Source: CAD feature listing. Evaluate the final solid. Frame: model axes, mm. A direction names the side the tool comes from. Round coordinates to 2 decimals unless told otherwise and drop trailing zeros. Loops run counter-clockwise (first coordinate to the right, second up) from the corner with the lowest first, then second, coordinate; pieces in that order, holes last.
Item 1: Access query for faces 1 (the flat face through (-9.2, 0, -11.938)), 2 (the flat face through (-8.7, 0, 0)), 3 (the flat face through (-0.039, 10, 1)), 4 (the flat face through (-5, 0, 11.43)). Directions: +Z, -Z, +X, -X, +Y, -Y. A direction counts if a zero-diameter tool reaches every point of the face in a straight line with its end or side. Return the directions, or none.
Item 2: Section query C-C on y = -6.5. Return loops of the section in (x, z).
Item 3: Section query A-A on z = 7. Return loops of the section in (x, y), then the cut area to 3 significant figures.
Item 4: Ray query, L1, parallel to Y at x = 0, z = 12.3 (3 decimals); L2, parallel to X at y = 0, z = 1.25 (3 decimals); L3, parallel to Y at x = 0, z = 3 (3 decimals). Return the intervals inside material, ascending.
Item 5: Section query B-B on y = 2.25. Return loops of the section in (x, z).
Item 6: Pull-direction query (Y, two-part tool) for faces 5 (the cylindrical face through (8.11, 6.33, -10.65)), 6 (the flat face through (-0.039, -10, 1)), 7 (the cylindrical face through (-0.96, -4.34, 12.72)); classes: released by +Y, released by -Y, zero draft, split by the parting line, or undercut.
Item 7: Section query D-D on x = 11.5. Return loops of the section in (y, z), then the cut area to 3 significant figures.
Item 8: First-contact query: P1, Ø1.5, axis at x = 5.5, z = -13, coming from the +Y side; P2, Ø5, axis at x = 15.5, y = 1, coming from the -Z side; P3, Ø3, axis at x = -2.5, y = 0.5, coming from the -Z side; P4, Ø4, axis at y = 9.5, z = -5, coming from the +X side. Flat tips, straight axial feed; report the tip coordinate or a pass-through.
Autodesk Inventor part; units mm, degrees
ref_plane "Work Plane1" through (0, 0, -9.398) normal (0, 0, 1) x (1, 0, 0)
ref_plane "Work Plane8" through (0, 12.4206, 0) normal (0, 1, 0) x (-1, 0, 0)
ref_plane "YZ Plane" through (0, 0, 0) normal (1, 0, 0) x (0, 1, 0)
sketch "Sketch2" plane through (0, 0, 0) normal (0, 0, 1) x (1, 0, 0)
  circle A0 centre (0, 0) radius 8.382
  dimension "d0" = 16.764
extrude "Extrusion1" add sketch "Sketch2" along normal blind 13.97
sketch "Sketch3" plane through (0, 0, 0) normal (0, 0, -1) x (-1, 0, 0)
  circle A0 centre (0, 0) radius 8.382
  circle A1 centre (0, 0) radius 8.89
  dimension "d3" = 17.78
extrude "Extrusion2" add sketch "Sketch3" along normal blind 17.018 contours A0 | A1
ref_plane "Work Plane1" through (0, 0, -9.398) normal (0, 0, 1) x (1, 0, 0)
sketch "Sketch4" plane through (0, 0, -9.398) normal (0, 0, 1) x (1, 0, 0)
  circle A0 centre (0, 0) radius 8.89
  circle A1 centre (0, 0) radius 10.287
  circle A2 centre (0, 0) radius 8.89
  dimension "d7" = 20.574
extrude "Extrusion3" add sketch "Sketch4" against normal blind 2.54
sketch "Sketch9" plane through (0, 0, -17.018) normal (0, 0, -1) x (-1, 0, 0)
  circle A0 centre (0, 0) radius 8.89
  circle A1 centre (0, 0) radius 6.985
  dimension "d40" = 13.97
extrude "Extrusion7" cut sketch "Sketch9" against normal blind 28.448 contours A1
sketch "Sketch10" plane through (0, 0, 13.97) normal (0, 0, 1) x (1, 0, 0)
  circle A0 centre (0, 0) radius 8.382
  circle A1 centre (0, 0) radius 4.445
  dimension "d43" = 8.89
extrude "Extrusion8" cut sketch "Sketch10" against normal up to surface (2.54 mm away) contours A1
sketch "Sketch12" plane through (0, 0, 0) normal (0, 1, 0) x (-1, 0, 0)
  line L0 (8.89, -17.018) -> (-8.89, -17.018)
  line L1 (-13.7704, -25.0461) -> (-13.7704, -36.5125) construction
  circle A0 centre (-16.256, -10.414) radius 1.524
  arc A1 (-16.256, -6.35) -> (-17.4864, -14.2873) centre (-16.256, -10.414) ccw
  line L2 (-16.256, -6.35) -> (-14.965, -6.35)
  line L3 (-14.965, -6.35) -> (-8.89, 0)
  line L4 (-8.89, 0) -> (-8.89, -9.398)
  line L5 (-8.89, -17.018) -> (-17.4864, -14.2873)
  line L6 (-8.89, 0) -> (-8.89, -17.018)
  point P0 (0, 0)
  dimension "d54" = 3.048
  dimension "d55" = 8.128
  dimension "d56" = 6.604
  dimension "d57" = 16.256
extrude "Extrusion9" add sketch "Sketch12" along normal mid plane 2.54
sketch "Sketch14" plane through (8.89, -1.27, -9.398) normal (-1, 0, 0) x (0, 0, 1)
  line L0 (0, 0) -> (0, 1.27)
  line L1 (0, 0) -> (9.398, 0)
  line L2 (9.398, 1.27) -> (9.398, 0)
  line L3 (9.398, 1.27) -> (0, 1.27)
  line L4 (-7.62, 2.54) -> (9.398, 2.54)
  line L5 (9.398, 2.54) -> (9.398, 0)
  line L6 (9.398, 0) -> (-7.62, 0)
  line L7 (-7.62, 0) -> (-7.62, 2.54)
extrude "Extrusion11" add sketch "Sketch14" along normal up to next contours L6 L7 L4 L5 L3 L0
sketch "Sketch15" plane through (0, 0, -17.018) normal (0, 0, -1) x (-1, 0, 0)
  arc A0 (6.8686, 1.27) -> (-6.8686, 1.27) centre (0, 0) ccw
  circle A1 centre (0, 0) radius 6.985
extrude "Extrusion12" cut sketch "Sketch15" against normal up to surface (28.448 mm away)
ref_plane "Work Plane8" through (0, 12.4206, 0) normal (0, 1, 0) x (-1, 0, 0)
sketch "Sketch16" plane through (0, 12.4206, 0) normal (0, 1, 0) x (-1, 0, 0)
  arc A0 (-3.7707, -10.668) -> (0.0393, -6.858) centre (0.0393, -10.668) ccw
  line L0 (-10.2083, -9.398) -> (10.287, -9.398)
  line L1 (10.287, -11.938) -> (-10.2083, -11.938)
  line L2 (-10.2083, -9.398) -> (10.287, -11.938) construction
  line L3 (-3.7707, -10.668) -> (-3.7707, 8.636)
  line L4 (-3.7707, 8.636) -> (0.0393, 8.636)
  line L5 (0.0393, 8.636) -> (0.0393, -6.858)
  line L6 (-8.382, 13.97) -> (8.382, 13.97)
  point P0 (0, 0)
  dimension "d63" = 7.62
  dimension "d65" = 3.81
  dimension "d66" = 5.334
extrude "Extrusion13" add sketch "Sketch16" against normal up to next
mirror "Mirror2" about plane through (0, 0, 0) normal (0, 1, 0) of "Extrusion13"
properties part number "Front Axle Body"
Data:
1. face 1: -Z, -X
1. face 2: +Z, -X
1. face 3: +Z, -X, +Y
1. face 4: -Z
2. outline: (-7.97, -11.94) - (-6.06, -11.94) - (-6.06, -17.02) - (-2.56, -17.02) - (-2.56, 11.43) - (2.56, 11.43) - (2.56, -17.02) - (6.06, -17.02) - (6.06, -11.94) - (7.97, -11.94) - (7.97, -9.4) - (6.06, -9.4) - (6.06, 0) - (5.29, 0) - (5.29, 13.97) - (-5.29, 13.97) - (-5.29, 0) - (-6.06, 0) - (-6.06, -9.4) - (-7.97, -9.4) - close
3. outline: (-0.04, -12.42) - (3.77, -12.42) - (3.77, -7.49) arc R8.38 ccw to (3.77, 7.49) - (3.77, 12.42) - (-0.04, 12.42) - (-0.04, 8.38) arc R8.38 ccw to (-0.04, -8.38) - close; hole circle Ø13.97 at (0, 0)
3. area: 100 mm2
4. L1: y = -8.382 to -4.445, 4.445 to 8.382
4. L2: x = -8.382 to -6.985, 6.985 to 8.382
4. L3: y = -12.421 to -6.985, 6.985 to 12.421
5. outline: (-10.04, -11.94) - (-8.6, -11.94) - (-8.6, -17.02) - (-6.61, -17.02) - (-6.61, 11.43) - (-3.83, 11.43) - (-3.83, 13.97) - (-8.07, 13.97) - (-8.07, 0) - (-8.6, 0) - (-8.6, -9.4) - (-10.04, -9.4) - close; (3.83, 11.43) - (6.61, 11.43) - (6.61, -17.02) - (8.6, -17.02) - (8.6, -11.94) - (10.04, -11.94) - (10.04, -9.4) - (8.6, -9.4) - (8.6, 0) - (8.07, 0) - (8.07, 13.97) - (3.83, 13.97) - close
6. face 5: released by +Y
6. face 6: zero draft
6. face 7: undercut
7. outline: (-1.27, -16.19) - (1.27, -16.19) - (1.27, -2.73) - (-1.27, -2.73) - close
7. area: 34.2 mm2
8. P1: stops at y = 7.51
8. P2: stops at z = -15.71
8. P3: passes through
8. P4: stops at x = 4.77
